Study the drawing (mm; zero at the part's minimum x, y, z) and answer. A direction names the side the tool comes from. Coordinates: 2 decimals unless noted, no trailing zeros. Write each loop counter-clockwise with the first axis right and the second up, starting at its lowest first coordinate (ties: lowest second). Pieces come first, ordered by that corner, then holes. Notation, with made-up numbers: (2, -15) - (11, -15) arc R38 ccw to (11, 24) - close; hole circle Ø4 at (-12.75, 39). An arc over 180 degrees is marked (long way). One line per item, written item: value.
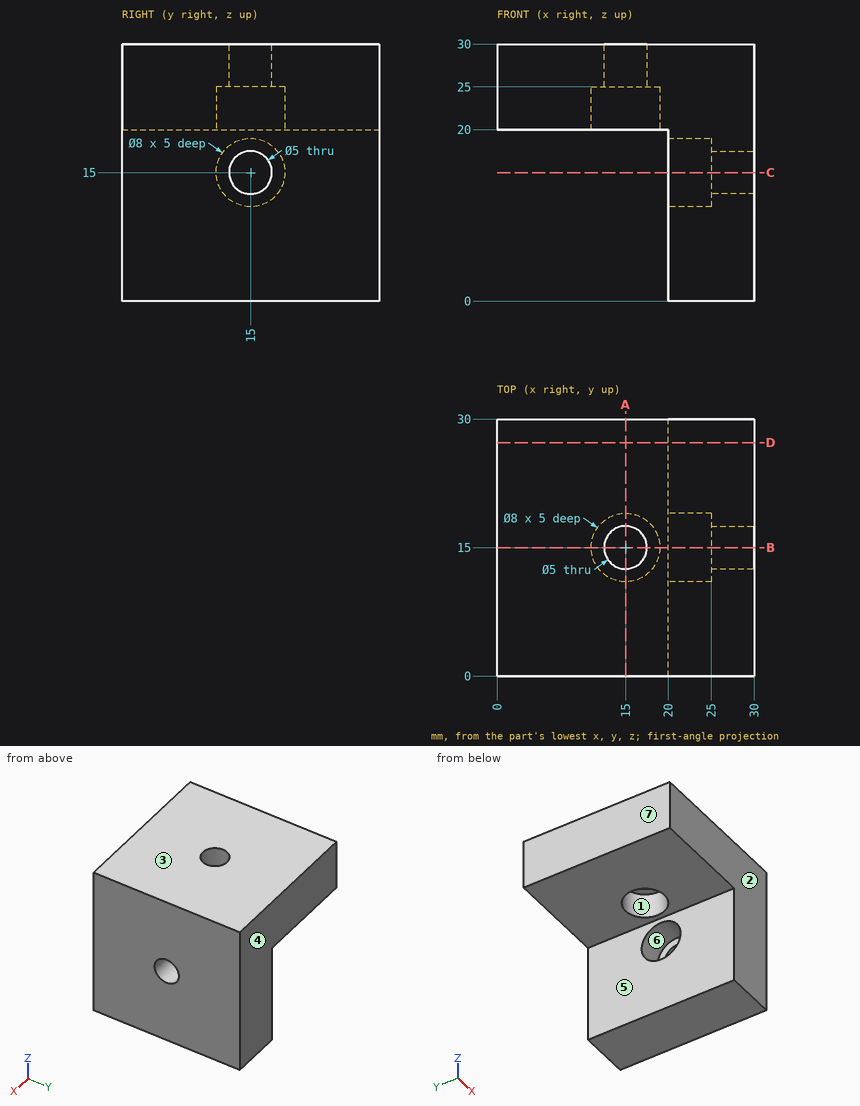
Item 1: Section B-B, the plane y = 15 is taken. Determine the outline of the cut face in (x, z).
Evaluation:
outline: (0, 20) - (11, 20) - (11, 25) - (12.5, 25) - (12.5, 30) - (0, 30) - close; (17.5, 25) - (19, 25) - (19, 20) - (20, 20) - (20, 19) - (25, 19) - (25, 17.5) - (30, 17.5) - (30, 30) - (17.5, 30) - close; (20, 0) - (30, 0) - (30, 12.5) - (25, 12.5) - (25, 11) - (20, 11) - close
Item 2: Given pin 1 (10 mm diameter, centred on x = 14.5, y = 7.5, fed in from -Z); pin 2 (16 mm diameter, centred on y = 8, z = 7, fed in from -X); pin 3 (6 mm diameter, centred on x = 15, y = 15, fed in from -Z), each flat-ended and moving along its own axis, determine where each tip first touches the part or whether it passes through.
Evaluation:
pin 1: stops at z = 20
pin 2: stops at x = 20
pin 3: stops at z = 25
Item 3: Section A-A, the plane x = 15 is taken. Determine the outline of the cut face in (y, z).
Evaluation:
outline: (0, 20) - (11, 20) - (11, 25) - (12.5, 25) - (12.5, 30) - (0, 30) - close; (17.5, 25) - (19, 25) - (19, 20) - (30, 20) - (30, 30) - (17.5, 30) - close
Item 4: Section C-C, the plane z = 15 is taken. Determine the outline of the cut face in (x, y), then the cut area to 3 significant figures.
Evaluation:
outline: (20, 0) - (30, 0) - (30, 12.5) - (25, 12.5) - (25, 11) - (20, 11) - close; (20, 19) - (25, 19) - (25, 17.5) - (30, 17.5) - (30, 30) - (20, 30) - close
area: 235 mm2
Item 5: Consider probe 1 along Y at (x, z) = (22.5, 15); probe 2 along Y at (x, z) = (27.1, 15); probe 3 along Z at (x, y) = (10.5, 28.75). Determine where each line is inside the solid, lowest interval first.
Evaluation:
probe 1: y = 0 to 11, 19 to 30
probe 2: y = 0 to 12.5, 17.5 to 30
probe 3: z = 20 to 30
Item 6: Which of the six approach directions +Z, -Z, +X, -X, +Y, -Y give full straight-line access (tool end or side, diameter ignored) to the marked faces 5, 6 and 7?
Evaluation:
face 5: -Z, -X, +Y, -Y
face 6: -X
face 7: +Z, -Z, -X, +Y, -Y
Item 7: Determine the mould class of the marked faces 1, 2, 3 and 4 for opening direction Y: +Y half, -Y half, draft (parallel to the pull), parting line (faces both ways), or undercut.
Evaluation:
face 1: undercut
face 2: -Y half
face 3: draft
face 4: +Y half
Item 8: Section D-D, the plane y = 27.25 is taken. Determine the outline of the cut face in (x, z).
Evaluation:
outline: (0, 20) - (20, 20) - (20, 0) - (30, 0) - (30, 30) - (0, 30) - close
